Autodesk Inventor part; units mm, degrees
ref_plane "Work Plane2" through (-25, -25, -8) normal (0, 0, -1) x (0, 1, 0)
ref_plane "YZ Plane" through (0, 0, 0) normal (1, 0, 0) x (0, 1, 0)
ref_plane "XZ Plane" through (0, 0, 0) normal (0, 1, 0) x (-1, 0, 0)
ref_plane "Work Plane1" through (0, 0, 0) normal (0, 0, 1) x (1, 0, 0)
sketch "Sketch1" plane through (0, 0, 0) normal (0, 0, 1) x (1, 0, 0)
  line L0 (9.1, -25) -> (9.1, -17.5)
  line L1 (9.1, -25) -> (25, -25)
  line L2 (25, -25) -> (25, -9.1)
  line L3 (17.5, -9.1) -> (25, -9.1)
  line L4 (17.5, -9.1) -> (17.5, -15.5)
  arc A0 (15.5, -17.5) -> (17.5, -15.5) centre (15.5, -15.5) ccw
  line L5 (15.5, -17.5) -> (9.1, -17.5)
  circle A1 centre (20, -20) radius 2.2989
  arc A2 (17.5, 15.5) -> (15.5, 17.5) centre (15.5, 15.5) ccw
  line L6 (-15.25, 17.25) -> (15.25, 17.25)
  line L7 (17.25, 15.25) -> (17.25, -15.25)
  line L8 (15.25, -17.25) -> (-15.25, -17.25)
  line L9 (-17.25, -15.25) -> (-17.25, 15.25)
  line L10 (-17.25, 17.25) -> (17.25, -17.25) construction
  line L11 (17.25, 17.25) -> (-17.25, -17.25) construction
  arc A3 (15.25, -17.25) -> (17.25, -15.25) centre (15.25, -15.25) ccw
  arc A4 (-17.25, -15.25) -> (-15.25, -17.25) centre (-15.25, -15.25) ccw
  arc A5 (-15.25, 17.25) -> (-17.25, 15.25) centre (-15.25, 15.25) ccw
  arc A6 (17.25, 15.25) -> (15.25, 17.25) centre (15.25, 15.25) ccw
  point P0 (0, 0)
  dimension "d0" = 34.5
  dimension "d1" = 34.5
  dimension "d2" = 2
ref_plane "Work Plane2" through (-25, -25, -8) normal (0, 0, -1) x (0, 1, 0)
extrude "Extrusion1" add sketch "Sketch1" against normal up to surface (8 mm away) contours L6 A6 L7 A3 L8 A4 L9 A5
sketch "Sketch2" plane through (-15.25, 17.25, 0) normal (0, 1, 0) x (1, 0, 0)
  arc A0 (22.85, 1.5) -> (24.35, 0) centre (24.35, 1.5) ccw
  line L0 (40.25, 0) -> (24.35, 0)
  line L1 (40.25, 0) -> (40.25, 8)
  line L2 (18.4, 8) -> (40.25, 8)
  line L3 (18.4, 8) -> (18.4, 5)
  line L4 (18.4, 5) -> (21.35, 5)
  arc A1 (22.85, 3.5) -> (21.35, 5) centre (21.35, 3.5) ccw
  line L5 (22.85, 3.5) -> (22.85, 1.5)
  circle A2 centre (27.75, 4) radius 1.75
  circle A3 centre (2.75, 4) radius 1.75
  arc A4 (6.15, 0) -> (7.65, 1.5) centre (6.15, 1.5) ccw
  line L6 (7.65, 1.5) -> (7.65, 3.5)
  arc A5 (9.15, 5) -> (7.65, 3.5) centre (9.15, 3.5) ccw
  line L7 (9.15, 5) -> (12.1, 5)
  line L8 (12.1, 5) -> (12.1, 8)
  line L9 (-9.75, 8) -> (12.1, 8)
  line L10 (-9.75, 0) -> (-9.75, 8)
  line L11 (6.15, 0) -> (-9.75, 0)
  line L12 (18.4, 5) -> (12.1, 5)
  line L13 (12.1, 5) -> (12.1, 8)
  line L14 (12.1, 8) -> (18.4, 8)
  line L15 (18.4, 8) -> (18.4, 5)
  line L16 (24.35, 0) -> (6.15, 0)
  circle A6 centre (27.75, 4) radius 1.4
  circle A7 centre (2.75, 4) radius 1.4
  point P0 (15.25, 0)
  dimension "d7" = 2.8
  dimension "d8" = 2.8
extrude "Extrusion2" cut sketch "Sketch2" against normal through all contours A0 L16 A4 L6 A5 L7 L12 L4 A1 L5 | A6 | A7
sketch "Sketch3" plane through (-6.1, 17.25, -5) normal (0, 0, 1) x (1, 0, 0)
  circle A0 centre (6.1, -17.25) radius 4.7436
pattern_circular "Circular Pattern1" count 2 over 90 about axis through (0, 0, -5) along (0, 0, 1) of "Extrusion2"
properties part number "10_Base_v0_plate"
Could you check a few things on this model? Use its own coordinates, in mm. A direction names the side the tool comes from. Give positions to 0.01 mm unless a question says otherwise; leave off trailing zeros. Order: outer loops, then holes, each group sorted by start corner. A loop starts at its lowest first (then second) coordinate and runs counter-clockwise, first axis right, second up.
Q1. Suppose I cut it at B-B, the plane x = -2. Write out the boundary of the cut face in (y, z).
Q2. For faces 1 (the cylindrical face through (9.37, -7.15, -4.57)), 2 (the flat face through (0, -15, -5)), 3 (the cylindrical face through (-11.165, 15.436, -4.421)), which set-ups out of +Z, -Z, +X, -X, +Y, -Y let a thin tool reach every point of the face, with its end or its side?
Q3. We'd pull the mould along Y, two halves only. Please class faces 4 (the cylindrical face through (-16.68, -16.65, -3.94)), 5 (the cylindrical face through (-12.49, -8.05, -0.43)), 6 (the flat face through (7.6, -12, -2)), 7 (the flat face through (-15, 0, -5)): +Y half, -Y half, draft (parallel to the pull), parting line (faces both ways), or undercut.
Q4. I'm going to push flat-ended pins straight in: P1, Ø4.5, axis at y = -12.5, z = -4, coming from the -X side; P2, Ø1.9, axis at x = -15.5, y = 1, coming from the +Z side; P3, Ø18.5, axis at x = -1.5, y = 3.5, coming from the +Z side; P4, Ø1.5, axis at x = 6.5, y = -11.5, coming from the +Z side. Where does each tip first touch, or does it pass through?
Q5. Suppose I cut it at A-A, the plane z = -2. Write out the boundary of the cut face in (x, y).
Q6. Suppose I cut it at C-C, the plane y = 8. Write out the boundary of the cut face in (x, z).
Q7. If I drill on line 1 along Z through (x, y) = (15.1, 12.5); line 2 along X through (y, z) = (9.5, -5.25); line 3 along Z through (x, y) = (2, -10.5), over which ranges is the centre line in solid material (lowest first)?
Solution:
1. outline: (-17.25, -8) - (17.25, -8) - (17.25, -5) - (13.48, -5) arc R1.4 cw to (11.52, -5) - (-11.52, -5) arc R1.4 cw to (-13.48, -5) - (-17.25, -5) - close
2. face 1: +Z, +X, -X
2. face 2: +Z, +Y, -Y
2. face 3: +Y, -Y
3. face 4: -Y half
3. face 5: undercut
3. face 6: draft
3. face 7: undercut
4. P1: stops at x = -17.25
4. P2: stops at z = -5
4. P3: stops at z = -0.01
4. P4: stops at z = -4.53
5. outline: (-17.25, -15.25) arc R2 ccw to (-15.25, -17.25) - (-7.6, -17.25) - (-7.6, -7.6) - (-17.25, -7.6) - close; (-17.25, 7.6) - (-7.6, 7.6) - (-7.6, 17.25) - (-15.25, 17.25) arc R2 ccw to (-17.25, 15.25) - close; (7.6, -17.25) - (15.25, -17.25) arc R2 ccw to (17.25, -15.25) - (17.25, -7.6) - (7.6, -7.6) - close; (7.6, 7.6) - (17.25, 7.6) - (17.25, 15.25) arc R2 ccw to (15.25, 17.25) - (7.6, 17.25) - close
6. outline: (-17.25, -8) - (17.25, -8) - (17.25, -0.48) - (8, -0.48) arc R1.5 ccw to (7.6, -1.5) - (7.6, -3.5) arc R1.5 cw to (6.1, -5) - (-6.1, -5) arc R1.5 cw to (-7.6, -3.5) - (-7.6, -1.5) arc R1.5 ccw to (-8, -0.48) - (-17.25, -0.48) - close; hole circle Ø2.8 at (-12.5, -4); hole circle Ø2.8 at (12.5, -4)
7. line 1: z = -8 to -5.4, -2.6 to 0
7. line 2: x = -17.25 to -13.13, -11.87 to 11.87, 13.13 to 17.25
7. line 3: z = -8 to -5
